from build123d import *

# Parameters (mm, degrees)
EXTRUDE_3_DEPTH     = 4
SKETCH_4_R          = 3
EXTRUDE_4_DEPTH     = 6
CUT_EXTRUDE_1_DEPTH = 2.5
SKETCH_7_R          = 3.65
CUT_EXTRUDE_2_DEPTH = 27.874709301
FILLET_1_R          = 1


with BuildPart() as part:
    # 草图1 → 凸台-拉伸3 (new body)
    with BuildSketch(Plane.XY):
        with BuildLine():
            Line((0, 5), (20, 5))
            ThreePointArc((20, 5), (25, 0), (20, -5))
            Line((20, -5), (0, -5))
            ThreePointArc((0, -5), (-5, 0), (0, 5))
        make_face()
    extrude(amount=EXTRUDE_3_DEPTH)

    # 草图4 → 凸台-拉伸4 (add)
    with BuildSketch(Plane.XY):
        with Locations((22, 0)):
            Circle(SKETCH_4_R)
    extrude(amount=-EXTRUDE_4_DEPTH)

    # 草图6 → 切除-拉伸1 (cut)
    with BuildSketch(Plane(origin=(0, 0, 0), x_dir=(-1, 0, 0), z_dir=(0, 0, -1))):
        with BuildLine():
            Line((-16.1875, 2.392664571), (-0.28515625, 3.638844035))
            ThreePointArc((-0.28515625, 3.638844035), (3.65, 0), (-0.28515625, -3.638844035))
            Line((-0.28515625, -3.638844035), (-16.1875, -2.392664571))
            ThreePointArc((-16.1875, -2.392664571), (-18.4, 0), (-16.1875, 2.392664571))
        make_face()
    extrude(amount=-CUT_EXTRUDE_1_DEPTH, mode=Mode.SUBTRACT)

    # 草图7 → 切除-拉伸2 (cut, through all)
    with BuildSketch(Plane(origin=(0, 0, 2.5), x_dir=(-1, 0, 0), z_dir=(0, 0, -1))):
        Circle(SKETCH_7_R)
    extrude(amount=-CUT_EXTRUDE_2_DEPTH, mode=Mode.SUBTRACT)

    # 圆角1
    fillet_1_edges = [part.edges().sort_by_distance(p)[0] for p in [
        (19, 0, -6),
    ]]
    fillet(fillet_1_edges, radius=FILLET_1_R)


solid = part.part
Source: CAD feature listing. Evaluate the final solid. Frame: model axes, mm. A direction names the side the tool comes from. Round coordinates to 2 decimals unless told otherwise and drop trailing zeros. Order: outer loops, then holes, each group sorted by start corner. A loop starts at its lowest first (then second) coordinate and runs counter-clockwise, first axis right, second up. Notation, with made-up numbers: (6, 53) - (13, 53) arc R20 cw to (13, 77) - close; hole circle Ø3 at (89, -16). An arc over 180 degrees is marked (long way). Use a Markdown table: item, result. Add a question column.
1. Set-up query: faces 1 (the flat face through (9, 0, 2.5)), 2 (the flat face through (14, 0, 4)). Return all of +Z, -Z, +X, -X, +Y, -Y with unobstructed straight access to the full face (end or side cutting, diameter ignored); none if empty.
2. Mould query, pull axis Y, two halves, no side actions, for faces 3 (the flat face through (10, -5, 2)), 4 (the flat face through (8.125, -3.024, 1.232)), 5 (the flat face through (10.2, 3.4, 0)), 6 (the flat face through (10, 5, 2)). Classes: +Y half, -Y half, draft (parallel to the pull), parting line (faces both ways), or undercut.
3. Section query B-B (z = -2.5). Return the cut outline in (x, y).
4. Section query A-A (x = 22). Return the cut outline in (y, z), then the cut area to 3 significant figures.
5. Section query C-C (x = 5). Return the cut outline in (y, z).
6. Line query: probe 1 along Y at (x, z) = (0, 2.8); probe 2 along X at (y, z) = (0, 3.3); probe 3 along Z at (x, y) = (18.75, 2.5). Output: solid intervals per line, ascending.
7. First-contact query: pin 1 (1.5 mm diameter, centred on y = -4, z = 2.5, fed in from +X); pin 2 (3.5 mm diameter, centred on x = 11, y = 0.5, fed in from -Z). Flat tips, straight axial feed; report the tip coordinate or a pass-through.
Derived:
| question | item | result |
|---|---|---|
| 1 | face 1 | -Z |
| 1 | face 2 | +Z, +X, -X, +Y, -Y |
| 2 | face 3 | -Y half |
| 2 | face 4 | undercut |
| 2 | face 5 | draft |
| 2 | face 6 | +Y half |
| 3 | outline | circle Ø6 at (22, 0) |
| 4 | outline | (-4.58, 0) - (-3, 0) - (-3, -5) arc R1 ccw to (-2, -6) - (2, -6) arc R1 ccw to (3, -5) - (3, 0) - (4.58, 0) - (4.58, 4) - (-4.58, 4) - close |
| 4 | area | 72.2 mm2 |
| 5 | outline | (-5, 0) - (-3.27, 0) - (-3.27, 2.5) - (3.27, 2.5) - (3.27, 0) - (5, 0) - (5, 4) - (-5, 4) - close |
| 6 | probe 1 | -5 to -3.65, 3.65 to 5 |
| 6 | probe 2 | -5 to -3.65, 3.65 to 25 |
| 6 | probe 3 | 0 to 4 |
| 7 | pin 1 | x = 23.8 |
| 7 | pin 2 | z = 2.5 |
